Could you check a few things on this model? Use its own coordinates, in mm. Face numbers are marked on the shaded views. Give positions to 0.01 mm unless a question says otherwise; leave off trailing zeros. Order: outer loops, then holes, each group sorted by start corner. A loop starts at its lowest first (then second) coordinate and runs counter-clockwise, first axis right, second up. Notation, with made-up numbers: (-24.75, -5) - (5.25, -5) arc R29 cw to (5.25, 20) - close; hole circle Ø11 at (51.5, 79.5). An arc over 180 degrees is marked (long way). Put each result on its own line as item: value.
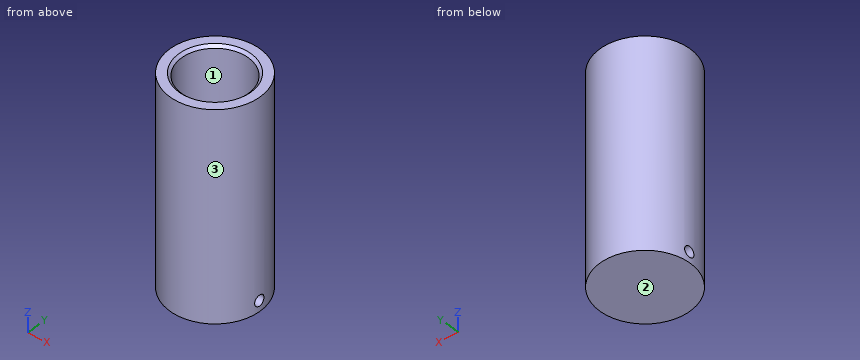
from build123d import *

# Parameters (mm, degrees)
F0_R      = 8.5
F1_DEPTH  = 2
F2_R      = 4
F3_DEPTH  = 20
F4_R      = 8.5
F4_R_2    = 6.3
F5_DEPTH  = 35
F6_SIZE   = 0.5
F7_SIZE   = 0.5
F8_R      = 2.5
F9_DEPTH  = 25
F10_R     = 1
F11_DEPTH = 12.5


with BuildPart() as f1:
    # F0 (on Top) → F1 (new body, symmetric)
    with BuildSketch(Plane.XY):
        Circle(F0_R)
    extrude(amount=F1_DEPTH, both=True)

    # F2 (on face) → F3 (join)
    with BuildSketch(Plane.XY.offset(2)):
        Circle(F2_R)
    extrude(amount=F3_DEPTH)

    # F4 (on face) → F5 (join)
    with BuildSketch(Plane.XY.offset(2)):
        Circle(F4_R)
        Circle(F4_R_2, mode=Mode.SUBTRACT)
    extrude(amount=F5_DEPTH)

    # F6
    f6_edges = [f1.edges().sort_by_distance(p)[0] for p in [
        (-4, 0, 22),
    ]]
    chamfer(f6_edges, length=F6_SIZE)

    # F7
    f7_edges = [f1.edges().sort_by_distance(p)[0] for p in [
        (-6.3, 0, 37),
    ]]
    chamfer(f7_edges, length=F7_SIZE)

    # F8 (on Top) → F9 (join)
    with BuildSketch(Plane.XY):
        Circle(F8_R)
    extrude(amount=F9_DEPTH)

    # F10 (on Right) → F11 (cut, symmetric)
    with BuildSketch(Plane.YZ):
        Circle(F10_R)
    extrude(amount=F11_DEPTH, both=True, mode=Mode.SUBTRACT)


solid = f1.part
1) I'm going to push flat-ended pins straight in: pin 1 (1.5 mm diameter, centred on x = 4.5, z = 27, fed in from +Y); pin 2 (4 mm diameter, centred on x = -3, z = 5.5, fed in from -Y); pin 3 (4 mm diameter, centred on x = 1, y = -1, fed in from +Z); pin 4 (1.6 mm diameter, centred on y = 0, z = 0, fed in from -X). Where does each tip first touch, or does it pass through?
Filled in:
pin 1: stops at y = 7.63
pin 2: stops at y = -8.44
pin 3: stops at z = 25
pin 4: passes through
2) Suppose I cut it at D-D, the plane z = 26.5. List the corners of the cut face in (x, y) for me.
Filled in:
outline: circle Ø17 at (0, 0); hole circle Ø12.6 at (0, 0)
3) If I drill on line 1 (Y direction, x = 0, z = 13.5); line 2 (Y direction, x = -2, z = 11); line 3 (Y direction, x = -2.75, z = 0), over which ranges is the centre line in solid material (lowest first)? Write a range as [from, to].
Filled in:
line 1: y = [-8.5, -6.3], [-4, 4], [6.3, 8.5]
line 2: y = [-8.26, -5.97], [-3.46, 3.46], [5.97, 8.26]
line 3: y = [-8.04, -1], [1, 8.04]
4) Suppose I cut it at C-C, the plane z = 6.5. List the corners of the cut face in (x, y) for me.
Filled in:
outline: circle Ø17 at (0, 0); circle Ø8 at (0, 0); hole circle Ø12.6 at (0, 0)
5) Suppose I cut it at A-A, the plane x = 0. List the corners of the cut face in (y, z) for me, and give its area (3 significant figures).
Filled in:
outline: (-8.5, -2) - (8.5, -2) - (8.5, 37) - (6.8, 37) - (6.3, 36.5) - (6.3, 2) - (4, 2) - (4, 21.5) - (3.5, 22) - (2.5, 22) - (2.5, 25) - (-2.5, 25) - (-2.5, 22) - (-3.5, 22) - (-4, 21.5) - (-4, 2) - (-6.3, 2) - (-6.3, 36.5) - (-6.8, 37) - (-8.5, 37) - close; hole circle Ø2 at (0, 0)
area: 393 mm^2
6) We'd pull the mould along Y, two halves only. Please class the marked faces 1, 2 and 3: pulls with the +Y half, pulls with the -Y half, needs draft (parallel to the pull), parting line crosses it, or undercut.
Filled in:
face 1: undercut
face 2: needs draft
face 3: parting line crosses it
7) Suppose I cut it at B-B, the plane y = 0. List the corners of the cut face in (x, z) for me, and give its area (4 significant figures).
Filled in:
outline: (-8.5, -2) - (8.5, -2) - (8.5, -1) - (-8.5, -1) - close; (-8.5, 1) - (8.5, 1) - (8.5, 37) - (6.8, 37) - (6.3, 36.5) - (6.3, 2) - (4, 2) - (4, 21.5) - (3.5, 22) - (2.5, 22) - (2.5, 25) - (-2.5, 25) - (-2.5, 22) - (-3.5, 22) - (-4, 21.5) - (-4, 2) - (-6.3, 2) - (-6.3, 36.5) - (-6.8, 37) - (-8.5, 37) - close
area: 362.5 mm^2
